Part model, mm, in its own coordinate system. A direction names the side the tool comes from. Round coordinates to 2 decimals unless told otherwise and drop trailing zeros. Loops run counter-clockwise (first coordinate to the right, second up) from the corner with the lowest first, then second, coordinate; pieces in that order, holes last.
1) Band-saw the part on C-C, the plane x = -115. Write the cut outline in (y, z).
2) Mould opens along Z. For faces 1 (the cylindrical face through (-56.553, -3.944, -32.066)), 2 (the flat face through (-570, 6, 40)), 3 (the cylindrical face through (-620.53, -3.09, -33.06)) say: +Z half, -Z half, draft (parallel to the pull), parting line (faces both ways), or undercut.
3) Band-saw the part on D-D, the plane x = -560.5. Write the cut outline in (y, z).
4) Drop flat-ended pins along their axis: P1, Ø1.5, axis at x = -547, z = 5, coming from the +Y side; P2, Ø18, axis at y = -4, z = 0, coming from the -X side; P3, Ø6, axis at x = -372, y = -13, coming from the +Z side; P4, Ø4, axis at x = -495.5, y = -9.5, coming from the +Z side. Give the stop position or say it passes through.
5) Band-saw the part on A-A, the plane z = 0. Write the cut outline in (x, y), then the cut area to 3 significant figures.
6) Band-saw the part on B-B, the plane x = -632. Write the cut outline in (y, z), then the cut area to 3 significant figures.
7) Probe line 1 (Z direction, x = -600, y = -4); line 2 (Z direction, x = -624, y = -3); line 3 (Y direction, x = -130, z = 0). List the from-to ranges inside material, lowest first.
8) 3-axis set-ups, long thin cutter, end or side, ignore diameter. For faces 4 (the cylindrical face through (-451.013, -3.944, -34.357)), 5 (the cylindrical face through (-104.468, 2.466, -2.681)), 6 (the cylindrical face through (-620.532, -0.737, -54.692)), 7 (the flat face through (-570, -13, 40)): which of +Z, -Z, +X, -X, +Y, -Y reach the whole face in a straight line?
from build123d import *

# Parameters (mm, degrees)
F2_DEPTH = 8
F3_R     = 15.05
F3_R_2   = 7
F4_DEPTH = 102.5
F5_R     = 15.05
F5_R_2   = 7
F6_DEPTH = 102.5
F9_DEPTH = 5


with BuildPart() as f2:
    # F1 (on Front) → F2 (new body)
    with BuildSketch(Plane.XZ):
        with BuildLine():
            Line((-155, 15), (-53.5, 15))
            Line((-53.5, 15), (-53.5, 24.8735827689))
            ThreePointArc((-53.5, 24.8735827689), (-56.4734852979, 31.9889247243), (-63.6256182283, 34.8727937409))
            Line((-63.6256182283, 34.8727937409), (-415.0965194239, 30.457330158))
            ThreePointArc((-415.0965194239, 30.457330158), (-450.5260994272, 34.2445631167), (-484.0628321732, 46.2814160866))
            Line((-484.0628321732, 46.2814160866), (-540.3854382, 74.4427191))
            ThreePointArc((-540.3854382, 74.4427191), (-562.1315056952, 82.3248989468), (-585.10679775, 85))
            Line((-585.10679775, 85), (-661.5, 85))
            ThreePointArc((-661.5, 85), (-668.5710678119, 82.0710678119), (-671.5, 75))
            Line((-671.5, 75), (-671.5, 55))
            Line((-671.5, 55), (-570, 55))
            Line((-570, 55), (-570, 25))
            Line((-570, 25), (-671.5, 25))
            Line((-671.5, 25), (-671.5, -25))
            Line((-671.5, -25), (-570, -25))
            Line((-570, -25), (-570, -55))
            Line((-570, -55), (-671.5, -55))
            Line((-671.5, -55), (-671.5, -75))
            ThreePointArc((-671.5, -75), (-668.5710678119, -82.0710678119), (-661.5, -85))
            Line((-661.5, -85), (-585.10679775, -85))
            ThreePointArc((-585.10679775, -85), (-562.1315056952, -82.3248989468), (-540.3854382, -74.4427191))
            Line((-540.3854382, -74.4427191), (-484.0628321732, -46.2814160866))
            ThreePointArc((-484.0628321732, -46.2814160866), (-450.5260994272, -34.2445631167), (-415.0965194239, -30.457330158))
            Line((-415.0965194239, -30.457330158), (-63.6256182283, -34.8727937409))
            ThreePointArc((-63.6256182283, -34.8727937409), (-56.4734852979, -31.9889247243), (-53.5, -24.8735827689))
            Line((-53.5, -24.8735827689), (-53.5, -15))
            Line((-53.5, -15), (-155, -15))
            Line((-155, -15), (-155, 15))
        make_face()
    extrude(amount=F2_DEPTH)

    # F3 (on face) → F4 (join)
    with BuildSketch(Plane.YZ.offset(-155)):
        with Locations((-4, 0)):
            Circle(F3_R)
        with Locations((-4, 0)):
            Circle(F3_R_2, mode=Mode.SUBTRACT)
    extrude(amount=F4_DEPTH)

    # F5 (on face) → F6 (join)
    with BuildSketch(Plane(origin=(-570, 0, 0), x_dir=(0, -1, 0), z_dir=(-1, 0, 0))):
        with Locations((4, 40)):
            Circle(F5_R)
        with Locations((4, 40)):
            Circle(F5_R_2, mode=Mode.SUBTRACT)
        with Locations((4, -40)):
            Circle(F5_R)
        with Locations((4, -40)):
            Circle(F5_R_2, mode=Mode.SUBTRACT)
    extrude(amount=F6_DEPTH)

    # F8 (on offset) → F9 (join)
    with BuildSketch(Plane(origin=(-646.5, 0, 0), x_dir=(0, -1, 0), z_dir=(-1, 0, 0))):
        with BuildLine():
            Line((25.6776695297, 61.7791627651), (8, 79.4568322948))
            Line((8, 79.4568322948), (8, 54.4568322948))
            ThreePointArc((8, 54.4568322948), (19, 40), (8, 25.5431677052))
            Line((8, 25.5431677052), (8, -25.5431677052))
            ThreePointArc((8, -25.5431677052), (19, -40), (8, -54.4568322948))
            Line((8, -54.4568322948), (8, -79.4568322948))
            Line((8, -79.4568322948), (25.6776695297, -61.7791627651))
            ThreePointArc((25.6776695297, -61.7791627651), (31.0969883128, -53.6685790446), (33, -44.1014932355))
            Line((33, -44.1014932355), (33, -10))
            Line((33, -10), (28, -10))
            Line((28, -10), (28, 10))
            Line((28, 10), (33, 10))
            Line((33, 10), (33, 44.1014932355))
            ThreePointArc((33, 44.1014932355), (31.0969883128, 53.6685790446), (25.6776695297, 61.7791627651))
        make_face()
    extrude(amount=F9_DEPTH)


solid = f2.part
Reported:
1. outline: (-8, -34.23) - (0, -34.23) - (0, -15) - (-2.77, -15) arc R15.05 ccw to (-2.77, 15) - (0, 15) - (0, 34.23) - (-8, 34.23) - (-8, 15) - (-5.23, 15) arc R15.05 ccw to (-5.23, -15) - (-8, -15) - close; hole circle Ø14 at (-4, 0)
2. face 1: -Z half
2. face 2: draft
2. face 3: undercut
3. outline: (-8, -81.93) - (0, -81.93) - (0, 81.93) - (-8, 81.93) - close
4. P1: stops at y = 0
4. P2: stops at x = -671.5
4. P3: passes through
4. P4: stops at z = 52.66
5. outline: (-671.5, -8) - (-651.5, -8) - (-651.5, -28) - (-646.5, -28) - (-646.5, -8) - (-155, -8) - (-155, 0) - (-671.5, 0) - close; (-155, -19.05) - (-52.5, -19.05) - (-52.5, -11) - (-155, -11) - close; (-155, 3) - (-52.5, 3) - (-52.5, 11.05) - (-155, 11.05) - close
5. area: 5,880 mm2
6. outline: (-8, -85) - (0, -85) - (0, -55) - (-2.77, -55) arc R15.05 ccw to (-2.77, -25) - (0, -25) - (0, 25) - (-2.77, 25) arc R15.05 ccw to (-2.77, 55) - (0, 55) - (0, 85) - (-8, 85) - (-8, 55) - (-5.23, 55) arc R15.05 ccw to (-5.23, 25) - (-8, 25) - (-8, -25) - (-5.23, -25) arc R15.05 ccw to (-5.23, -55) - (-8, -55) - close; hole circle Ø14 at (-4, -40); hole circle Ø14 at (-4, 40)
6. area: 1,990 mm2
7. line 1: z = -85 to -47, -33 to 33, 47 to 85
7. line 2: z = -85 to -46.93, -33.07 to 33.07, 46.93 to 85
7. line 3: y = -19.05 to -11, 3 to 11.05
8. face 4: -Z, +Y, -Y
8. face 5: +X
8. face 6: none
8. face 7: +Z, -Z, +X, -Y
